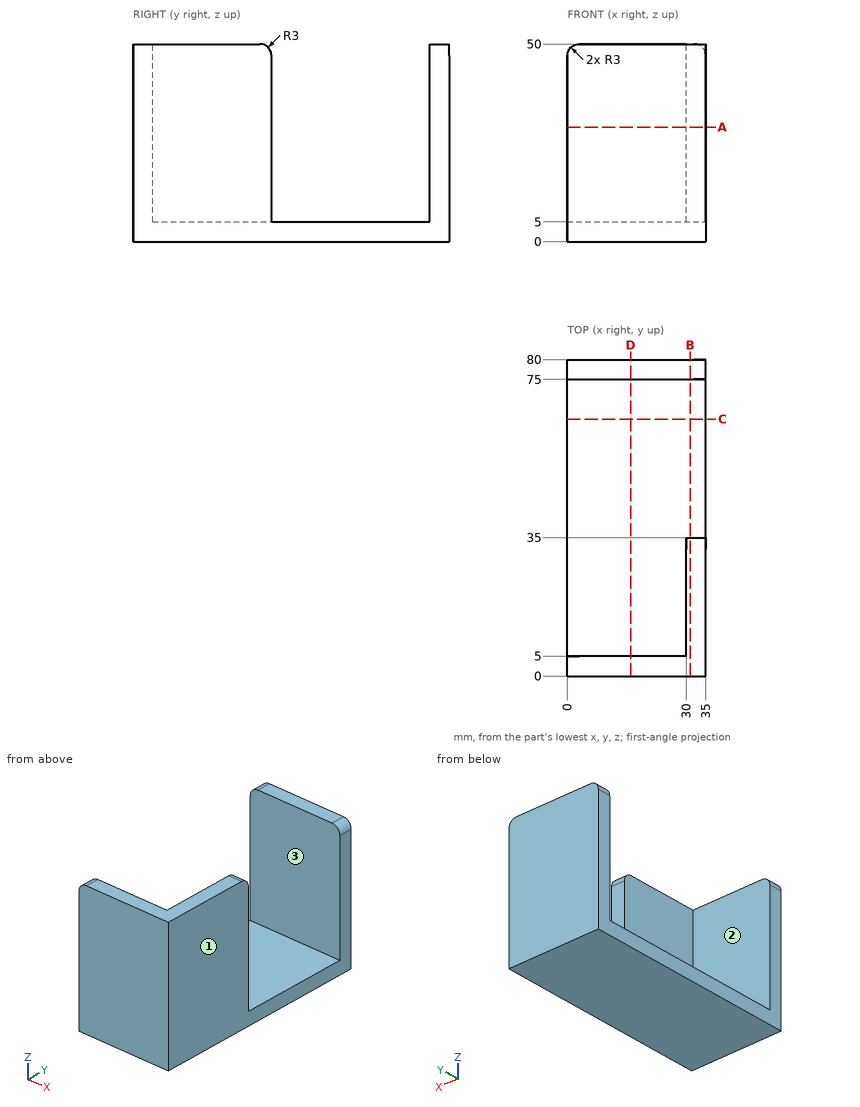
Drawing for the job (mm, zero at the part's lowest x, y, z). A direction names the side the tool comes from. Coordinates: 2 decimals unless noted, no trailing zeros. Write each loop counter-clockwise with the first axis right and the second up, starting at its lowest first coordinate (ties: lowest second). Pieces come first, ordered by that corner, then holes. Notation, with made-up numbers: (0, 85.5) -> (16, 85.5) arc R34 ccw to (16, 124.5) -> close; hole circle Ø2 at (27.5, 46.25). An arc over 180 degrees is marked (long way). One line per item, written item: value. Start each with the question number.
1) Flat gauge pins, fed straight in: pin 1 Ø9 at (y, z) = (14, 36) entering from -X; pin 2 Ø8 at (x, y) = (9.5, 17.5) entering from +Z; pin 3 Ø4 at (y, z) = (71.5, 16.5) entering from -X. Where does each tip first touch, or does it go through?
2) Slice it at A-A on z = 29. Write the cut outline in (x, y).
3) Slice it at C-C on y = 65. Write the cut outline in (x, z).
4) Slice it at D-D on x = 16. Write the cut outline in (y, z), then the cut area to 3 significant figures.
5) Probe probe 1 along Y at (x, z) = (2, 34.5); probe 2 along Z at (x, y) = (27.5, 71); probe 3 along X at (y, z) = (34, 24). List the from-to ranges inside material, lowest first.
6) Which spindle directions (+Z, -Z, +X, -X, +Y, -Y) get a long thin tool onto all of the face, cutting with end or side? Do the marked faces 1, 2 and 3. Say none if no direction does.
7) Slice it at B-B on x = 31. Write the cut outline in (y, z).
Answers follow:
1. pin 1: x = 30
1. pin 2: z = 5
1. pin 3: through
2. outline: (0, 0) -> (35, 0) -> (35, 35) -> (30, 35) -> (30, 5) -> (0, 5) -> close; (0, 75) -> (35, 75) -> (35, 80) -> (0, 80) -> close
3. outline: (0, 0) -> (35, 0) -> (35, 5) -> (0, 5) -> close
4. outline: (0, 0) -> (80, 0) -> (80, 50) -> (75, 50) -> (75, 5) -> (5, 5) -> (5, 50) -> (0, 50) -> close
4. area: 850 mm2
5. probe 1: 0 to 5, 75 to 80
5. probe 2: 0 to 5
5. probe 3: 30 to 35
6. face 1: +Z, -Z, +X, +Y, -Y
6. face 2: +Z, -X
6. face 3: +Z, +X, -X
7. outline: (0, 0) -> (80, 0) -> (80, 50) -> (75, 50) -> (75, 5) -> (35, 5) -> (35, 47) arc R3 ccw to (32, 50) -> (0, 50) -> close
